CAD build for the part. Positions are in the model's coordinates, mm. A direction names the side the tool comes from. Give positions to 0.01 mm unless a question says otherwise; leave off trailing zeros. Loops run counter-clockwise (first coordinate to the right, second up) from the corner with the lowest first, then second, coordinate; pieces in that order, holes last. Notation, with made-up numbers: (83, 3.25) -> (121, 3.25) arc R16 cw to (121, 21.25) -> close; hole circle Ø5 at (37, 35.5). An arc over 180 degrees is marked (long way). Use one line per item in the form item = value.
```python
from build123d import *

# Parameters (mm, degrees)
EXTRUDE1_DEPTH = 101.6


with BuildPart() as part:
    # Sketch1 → Extrude1 (new body)
    with BuildSketch(Plane(origin=(0, 0, 0), x_dir=(1, 0, 0), z_dir=(0, 1, 0))):
        Polygon((0, 36.981224411), (0, 0), (42.615353822, 0), (51.897733448, -10.30089681), (80.325021053, -10.30089681), (89.607400679, 0), (132.222754501, 0), (132.222754501, 36.981224411), align=None)
    extrude(amount=-EXTRUDE1_DEPTH)


solid = part.part
```
1. Cut at C-C, the plane z = 7.5. Write the cut outline in (x, y), then the cut area to 3 significant figures.
Result sheet:
outline = (49.37, -101.6) -> (82.85, -101.6) -> (82.85, 0) -> (49.37, 0) -> close
area = 3,400 mm^2
2. Drill centre lines: line 1 (Z direction, x = 100, y = -46); line 2 (X direction, y = -13, z = 8); line 3 (X direction, y = -38.5, z = 6.5). Where is each one in solid material? Low to high.
Result sheet:
line_1 = -36.98 to 0
line_2 = 49.82 to 82.4
line_3 = 48.47 to 83.75
3. Cut at B-B, the plane x = 22. Write the cut outline in (y, z), then the cut area to 3 significant figures.
Result sheet:
outline = (-101.6, -36.98) -> (0, -36.98) -> (0, 0) -> (-101.6, 0) -> close
area = 3,760 mm^2
4. Tool access for faces 1 (the flat face through (21, -50, 0)), 2 (the flat face through (111, -50, 0)), 3 (the flat face through (66, -50, 10.301)): list every direction of +Z, -Z, +X, -X, +Y, -Y with a clear straight run to the whole face (end or side of a thin tool).
Result sheet:
face_1 = +Z, -X, +Y, -Y
face_2 = +Z, +X, +Y, -Y
face_3 = +Z, +X, -X, +Y, -Y
5. Drop a flat-ended pin along its axis: P1, Ø13, axis at x = 120, y = -52, coming from the +Z side. Give the stop position or say it passes through.
Result sheet:
P1 = 0
6. Cut at A-A, the plane y = -46. Write the cut outline in (x, z).
Result sheet:
outline = (0, -36.98) -> (132.22, -36.98) -> (132.22, 0) -> (89.61, 0) -> (80.33, 10.3) -> (51.9, 10.3) -> (42.62, 0) -> (0, 0) -> close
